Work out the finished part from the listing and answer in its coordinate system (mm). Round coordinates to 2 decimals unless told otherwise and drop trailing zeros.
1. A flat-ended cylindrical pin translates along its axis: pin 1 Ø4.5 at (x, z) = (-139.41, 57.57) entering from +Y. Find the tip coordinate at first contact, or state that the pin passes through.
2. Find section A-A (y = 3). Count the separate pieces of the cut face and the enclosed holes in it, and give its area (3 significant figures).
3. Straight lines are drawn through the part: probe 1 along X at (y, z) = (5, 58.5); probe 2 along Z at (x, y) = (-168, 5.25); probe 3 along Z at (x, y) = (-169.5, 3.5). For each, find the intervals that lie inside material, in ascending order.
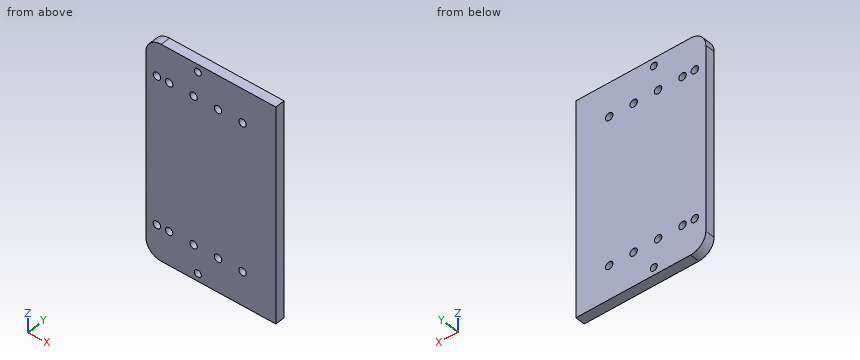
```python
from build123d import *

# Parameters (mm, degrees)
SKETCH1_W           = 85
SKETCH1_H           = 140
BOSS_EXTRUDE1_DEPTH = 6.35
FILLET1_R           = 10
SKETCH2_R           = 2.425
CUT_EXTRUDE1_DEPTH  = 6.35
SKETCH3_R           = 2.25
CUT_EXTRUDE2_DEPTH  = 10


with BuildPart() as part:
    # Sketch1 → Boss-Extrude1 (new body)
    with BuildSketch(Plane(origin=(0, 0, 0), x_dir=(1, 0, 0), z_dir=(0, 1, 0))):
        with Locations((-160.106308554, -105.56948084)):
            Rectangle(SKETCH1_W, SKETCH1_H)
    extrude(amount=BOSS_EXTRUDE1_DEPTH)

    # Fillet1
    fillet1_edges = [part.edges().sort_by_distance(p)[0] for p in [
        (-202.606308554, 3.175, 35.56948084),
        (-202.606308554, 3.175, 175.56948084),
    ]]
    fillet(fillet1_edges, radius=FILLET1_R)

    # Sketch2 → Cut-Extrude1 (cut)
    with BuildSketch(Plane.XZ):
        with Locations((-139.406308554, 57.56948084)):
            Circle(SKETCH2_R)
        with Locations((-155.406308554, 57.56948084)):
            Circle(SKETCH2_R)
        with Locations((-171.406308554, 57.56948084)):
            Circle(SKETCH2_R)
        with Locations((-187.406308554, 57.56948084)):
            Circle(SKETCH2_R)
        with Locations((-195.406308554, 57.56948084)):
            Circle(SKETCH2_R)
        with Locations((-139.406308554, 153.56948084)):
            Circle(SKETCH2_R)
        with Locations((-155.406308554, 153.56948084)):
            Circle(SKETCH2_R)
        with Locations((-171.406308554, 153.56948084)):
            Circle(SKETCH2_R)
        with Locations((-187.406308554, 153.56948084)):
            Circle(SKETCH2_R)
        with Locations((-195.406308554, 153.56948084)):
            Circle(SKETCH2_R)
    extrude(amount=-CUT_EXTRUDE1_DEPTH, mode=Mode.SUBTRACT)

    # Sketch3 → Cut-Extrude2 (cut)
    with BuildSketch(Plane.XZ):
        with Locations((-168.606308554, 170.56948084)):
            Circle(SKETCH3_R)
        with Locations((-168.606308554, 40.56948084)):
            Circle(SKETCH3_R)
    extrude(amount=-CUT_EXTRUDE2_DEPTH, mode=Mode.SUBTRACT)


solid = part.part
```
Worked answers:
1. pin 1: passes through
2. separate pieces: 1
2. enclosed holes: 12
2. area: 11,600 mm2
3. probe 1: x = -202.61 to -197.65, -193.17 to -189.65, -185.17 to -173.65, -169.17 to -157.65, -153.17 to -141.65, -137.17 to -117.61
3. probe 2: z = 35.57 to 38.4, 42.74 to 168.4, 172.74 to 175.57
3. probe 3: z = 35.57 to 38.5, 42.63 to 56.07, 59.07 to 152.07, 155.07 to 168.5, 172.63 to 175.57
